Check sheet for the modelled part. Datum: model origin and axes. Units: mm. A direction names the side the tool comes from. Round coordinates to 2 decimals unless told otherwise and drop trailing zeros. Loops run counter-clockwise (first coordinate to the right, second up) from the corner with the lowest first, then second, coordinate; pieces in that order, holes last. Notation, with made-up numbers: (-15, 18.25) -> (35, 18.25) arc R18 cw to (35, 43.25) -> close; hole circle Ø9 at (38, 77.5). An arc over 180 degrees is marked (long way). Return JSON: item names as keys, results as strings.
from build123d import *

# Parameters (mm, degrees)
SKETCH1_R                 = 33.9725
BOSS_EXTRUDE2_DEPTH       = 6.35
SKETCH2_R                 = 17.145
BOSS_EXTRUDE3_DEPTH       = 6.985
SKETCH3_W                 = 40.64
SKETCH3_H                 = 40.64
BOSS_EXTRUDE4_DEPTH       = 7.7724
SKETCH4_R                 = 10.2616
CUT_EXTRUDE1_DEPTH        = 22.1074
F_6_32_TAPPED_HOLE1_D     = 2.7051
F_6_32_TAPPED_HOLE1_DEPTH = 9.398
F_6_32_TAPPED_HOLE1_TIP   = 0.81269403
SKETCH8_R                 = 12.6238
SKETCH8_R_2               = 10.2616
BOSS_EXTRUDE5_DEPTH       = 6.7564


with BuildPart() as part:
    # Sketch1 → Boss-Extrude2 (new body)
    with BuildSketch(Plane.XY):
        Circle(SKETCH1_R)
    extrude(amount=BOSS_EXTRUDE2_DEPTH)

    # Sketch2 → Boss-Extrude3 (add)
    with BuildSketch(Plane(origin=(0, 0, 0), x_dir=(-1, 0, 0), z_dir=(0, 0, -1))):
        Circle(SKETCH2_R)
    extrude(amount=BOSS_EXTRUDE3_DEPTH)

    # Sketch3 → Boss-Extrude4 (add)
    with BuildSketch(Plane.XY.offset(6.35)):
        Rectangle(SKETCH3_W, SKETCH3_H)
    extrude(amount=BOSS_EXTRUDE4_DEPTH)

    # Sketch4 → Cut-Extrude1 (cut, through all)
    with BuildSketch(Plane.XY.offset(14.1224)):
        Circle(SKETCH4_R)
    extrude(amount=-CUT_EXTRUDE1_DEPTH, mode=Mode.SUBTRACT)

    # #6-32 Tapped Hole1
    with Locations(Plane.XY.offset(14.1224)):
        with Locations((-13.335, 13.335), (13.335, 13.335), (13.335, -13.335), (-13.335, -13.335)):
            Hole(F_6_32_TAPPED_HOLE1_D / 2, depth=F_6_32_TAPPED_HOLE1_DEPTH)
            with Locations((0, 0, -(F_6_32_TAPPED_HOLE1_DEPTH + F_6_32_TAPPED_HOLE1_TIP / 2))):  # 118° drill point
                Cone(0, F_6_32_TAPPED_HOLE1_D / 2, F_6_32_TAPPED_HOLE1_TIP, mode=Mode.SUBTRACT)

    # Sketch8 → Boss-Extrude5 (add)
    with BuildSketch(Plane.XY.offset(14.1224)):
        Circle(SKETCH8_R)
        Circle(SKETCH8_R_2, mode=Mode.SUBTRACT)
    extrude(amount=BOSS_EXTRUDE5_DEPTH)


solid = part.part
Q1. Draft check along Y on faces 5 (the flat face through (-20.32, 0, 10)), 6 (the flat face through (0, -20.32, 10)), 7 (the cylindrical face through (12.086, -13.853, 9.358)), 8 (the cylindrical face through (12.086, 12.817, 9.358)). Enter one of: released by +Y, released by -Y, zero draft, split by the parting line, or undercut.
Results list:
{"face 5": "zero draft", "face 6": "released by -Y", "face 7": "undercut", "face 8": "undercut"}
Q2. Go/stop test with flat-tipped pins: pin 1 (12.5 mm diameter, centred on x = 0, y = 0, fed in from +Z); pin 2 (6 mm diameter, centred on y = 9.5, z = 11.5, fed in from -X); pin 3 (2.5 mm diameter, centred on x = -13.335, y = 13.335, fed in from +Z); pin 4 (2 mm diameter, centred on y = 14, z = 6, fed in from +X). Record where each tip stops, or that it passes through.
Results list:
{"pin 1": "through", "pin 2": "x = -20.32", "pin 3": "z = 4.66", "pin 4": "x = 31.39"}
Q3. Material ranges on line 1 (Y direction, x = 0, z = 18.25); line 2 (Y direction, x = 0, z = 4.25); line 3 (Z direction, x = 1.5, y = 21), recorded low to high.
Results list:
{"line 1": "-12.62 to -10.26, 10.26 to 12.62", "line 2": "-33.97 to -10.26, 10.26 to 33.97", "line 3": "0 to 6.35"}
Q4. Section check D-D (y = 19). Record the boundary of the cut face in (x, z), then the cut area to 3 significant figures.
Results list:
{"outline": "(-28.16, 0) -> (28.16, 0) -> (28.16, 6.35) -> (20.32, 6.35) -> (20.32, 14.12) -> (-20.32, 14.12) -> (-20.32, 6.35) -> (-28.16, 6.35) -> close", "area": "674 mm^2"}
Q5. Section check C-C (z = 18). Record the boundary of the cut face in (x, y).
Results list:
{"outline": "circle Ø25.25 at (0, 0); hole circle Ø20.52 at (0, 0)"}
Q6. Tool access check on faces 1 (the flat face through (20.32, 0, 10)), 2 (the flat face through (-16, 8, 0)), 3 (the flat face through (0, 20.32, 10)), 4 (the flat face through (-9.3, 9.3, 14.122)). Record the directions out of +Z, -Z, +X, -X, +Y, -Y that give a thin tool (end or side, any length) a straight path to the whole face; none if there is none.
Results list:
{"face 1": "+Z, +X, +Y, -Y", "face 2": "-Z", "face 3": "+Z, +X, -X, +Y", "face 4": "+Z"}
